from build123d import *

# Parameters (mm, degrees)
ESQUISSE1_W             = 77
ESQUISSE1_H             = 73.5
ESQUISSE1_R             = 1.5
BOSS_EXTRU_1_DEPTH      = 3
ESQUISSE45_W            = 54.5
ESQUISSE45_H            = 3
BOSS_EXTRU_2_DEPTH      = 3
ESQUISSE46_W            = 54.5
ESQUISSE46_H            = 3
BOSS_EXTRU_3_DEPTH      = 25
CONG_1_R                = 5
ESQUISSE47_R            = 1.5
ENL_V_MAT_EXTRU_2_DEPTH = 25


with BuildPart() as part:
    # Esquisse1 → Boss.-Extru.1 (new body)
    with BuildSketch(Plane.XY):
        Rectangle(ESQUISSE1_W, ESQUISSE1_H)
        with Locations((30, 32.15)):
            Circle(ESQUISSE1_R, mode=Mode.SUBTRACT)
        with Locations((30, -32.85)):
            Circle(ESQUISSE1_R, mode=Mode.SUBTRACT)
        with Locations((-30, -32.85)):
            Circle(ESQUISSE1_R, mode=Mode.SUBTRACT)
        with Locations((-30, 32.15)):
            Circle(ESQUISSE1_R, mode=Mode.SUBTRACT)
    extrude(amount=BOSS_EXTRU_1_DEPTH)

    # Esquisse45 → Boss.-Extru.2 (add)
    with BuildSketch(Plane(origin=(0, 36.75, 0), x_dir=(1, 0, 0), z_dir=(0, 1, 0))):
        with Locations((0, -1.5)):
            Rectangle(ESQUISSE45_W, ESQUISSE45_H)
    extrude(amount=BOSS_EXTRU_2_DEPTH)

    # Esquisse46 → Boss.-Extru.3 (add)
    with BuildSketch(Plane.XY.offset(3)):
        with Locations((0, 38.25)):
            Rectangle(ESQUISSE46_W, ESQUISSE46_H)
    extrude(amount=BOSS_EXTRU_3_DEPTH)

    # Congé1
    cong_1_edges = [part.edges().sort_by_distance(p)[0] for p in [
        (0, 39.75, 0),
    ]]
    fillet(cong_1_edges, radius=CONG_1_R)

    # Esquisse47 → Enlèv. mat.-Extru.2 (cut)
    with BuildSketch(Plane(origin=(0, 39.75, 0), x_dir=(1, 0, 0), z_dir=(0, 1, 0))):
        with Locations(Location((0, -24.742583048, 0), (0, 0, 270))):
            Circle(ESQUISSE47_R)
    extrude(amount=-ENL_V_MAT_EXTRU_2_DEPTH, mode=Mode.SUBTRACT)


solid = part.part
Input: part model. Units: mm. Frame: model coordinates. A direction names the side the tool comes from. Coordinates: 2 decimals unless noted, no trailing zeros. Loops run counter-clockwise (first coordinate to the right, second up) from the corner with the lowest first, then second, coordinate; pieces in that order, holes last.
(1) Section C-C on z = 2. Return the cut outline in (x, y).
(2) Section D-D on x = 0. Return the cut outline in (y, z), then the cut area to 3 significant figures.
(3) Pull-direction query (Y, two-part tool) for faces 6 (the face through (27.25, 38, 14)), 7 (the face through (0, 39.75, 16)), 8 (the face through (28.81, -33.76, 1.48)); classes: released by +Y, released by -Y, zero draft, split by the parting line, or undercut.
(4) Set-up query: faces 1 (the face through (-1, 1, 3)), 2 (the face through (0.54, 38.25, 1.43)), 3 (the face through (-33, 36.75, 2)), 4 (the face through (-1, -36.75, 1)), 5 (the face through (33, 36.75, 2)). Return all of +Z, -Z, +X, -X, +Y, -Y with unobstructed straight access to the full face (end or side cutting, diameter ignored); none if empty.
(5) Section B-B on x = -30. Return the cut outline in (y, z).
(6) Material intervals for probe 1 along Y at (x, z) = (-30, 1.55); probe 2 along Z at (x, y) = (21, -6); probe 3 along Y at (x, z) = (3.5, 22.25), sorted ascending.
(7) First-contact query: pin 1 Ø12 at (x, y) = (-11.5, -20) entering from +Z; pin 2 Ø4 at (x, z) = (12, 24.5) entering from -Y; pin 3 Ø2 at (x, z) = (33, 1.5) entering from +Y. Flat tips, straight axial feed; report the tip coordinate or a pass-through.
(8) Section A-A on y = -32.85. Return the cut outline in (x, z), then the cut area to 3 significant figures.
Data:
1. outline: (-38.5, -36.75) - (38.5, -36.75) - (38.5, 36.75) - (27.25, 36.75) - (27.25, 38.75) - (-27.25, 38.75) - (-27.25, 36.75) - (-38.5, 36.75) - close; hole circle Ø3 at (-30, -32.85); hole circle Ø3 at (-30, 32.15); hole circle Ø3 at (30, -32.85); hole circle Ø3 at (30, 32.15)
2. outline: (-36.75, 0) - (34.75, 0) arc R5 ccw to (39.75, 5) - (39.75, 23.24) - (36.75, 23.24) - (36.75, 3) - (-36.75, 3) - close; (36.75, 26.24) - (39.75, 26.24) - (39.75, 28) - (36.75, 28) - close
2. area: 290 mm2
3. face 6: zero draft
3. face 7: released by +Y
3. face 8: undercut
4. face 1: +Z, +X, -X, -Y
4. face 2: -Z, +X, -X, +Y
4. face 3: +Z, -Z, -X, +Y
4. face 4: +Z, -Z, +X, -X, -Y
4. face 5: +Z, -Z, +X, +Y
5. outline: (-36.75, 0) - (-34.35, 0) - (-34.35, 3) - (-36.75, 3) - close; (-31.35, 0) - (30.65, 0) - (30.65, 3) - (-31.35, 3) - close; (33.65, 0) - (34.75, 0) arc R5 ccw to (36.75, 0.42) - (36.75, 3) - (33.65, 3) - close
6. probe 1: y = -36.75 to -34.35, -31.35 to 30.65, 33.65 to 36.75
6. probe 2: z = 0 to 3
6. probe 3: y = 36.75 to 39.75
7. pin 1: stops at z = 3
7. pin 2: stops at y = 36.75
7. pin 3: stops at y = 36.75
8. outline: (-38.5, 0) - (-31.5, 0) - (-31.5, 3) - (-38.5, 3) - close; (-28.5, 0) - (28.5, 0) - (28.5, 3) - (-28.5, 3) - close; (31.5, 0) - (38.5, 0) - (38.5, 3) - (31.5, 3) - close
8. area: 213 mm2
